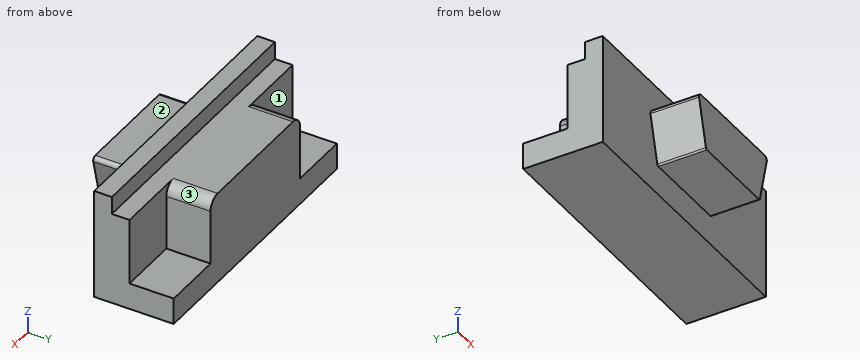
from build123d import *

# Parameters (mm, degrees)
SKETCH008_W          = 30.8
SKETCH008_H          = 12.5
PAD006_DEPTH         = 2
SKETCH009_W          = 30.8
SKETCH009_H          = 10.5
PAD007_DEPTH         = 2
PAD067_DEPTH         = 5
PAD115_DEPTH         = 5.5
BODY_PLACEMENT_ANGLE = 180


with BuildPart() as part:
    # Sketch008 → Pad006 (new body)
    with BuildSketch(Plane(origin=(0, 3, 0), x_dir=(-1, 0, 0), z_dir=(0, 1, 0))):
        with Locations((0, 6.25)):
            Rectangle(SKETCH008_W, SKETCH008_H)
    extrude(amount=-PAD006_DEPTH)

    # Sketch009 → Pad007 (join)
    with BuildSketch(Plane.XZ.offset(-1)):
        with Locations((0, 5.25)):
            Rectangle(SKETCH009_W, SKETCH009_H)
    extrude(amount=PAD007_DEPTH)

    # Sketch010 → Pad067 (join)
    with BuildSketch(Plane.XZ.offset(1)):
        with BuildLine():
            Line((15.4, 0), (15.4, 3))
            Line((15.4, 3), (8.45, 3))
            Line((8.45, 3), (8.45, 9.167398))
            ThreePointArc((8.45, 9.167398), (8.05969, 10.10969), (7.117398, 10.5))
            Line((7.117398, 10.5), (-7.117398, 10.5))
            ThreePointArc((-7.117398, 10.5), (-8.05969, 10.10969), (-8.45, 9.167398))
            Line((-8.45, 9.167398), (-8.45, 3))
            Line((-8.45, 3), (-15.4, 3))
            Line((-15.4, 3), (-15.4, 0))
            Line((-15.4, 0), (15.4, 0))
        make_face()
    extrude(amount=PAD067_DEPTH)

    # Sketch094 → Pad115 (join)
    with BuildSketch(Plane(origin=(0, 3, 0), x_dir=(-1, 0, 0), z_dir=(0, 1, 0))):
        with BuildLine():
            Line((-6, 9.18), (6, 9.18))
            ThreePointArc((6.390856, 8.68), (6.31732, 9.025285), (6, 9.18))
            Line((6.390856, 8.68), (5.098578, 3.485231))
            ThreePointArc((4.9, 3.33), (5.026026, 3.373413), (5.098578, 3.485231))
            Line((4.9, 3.33), (-4.9, 3.33))
            ThreePointArc((-5.098578, 3.485231), (-5.026026, 3.373413), (-4.9, 3.33))
            Line((-5.098578, 3.485231), (-6.390856, 8.68))
            ThreePointArc((-6, 9.18), (-6.31732, 9.025285), (-6.390856, 8.68))
        make_face()
    extrude(amount=PAD115_DEPTH)


with BuildPart() as part_1:
    # Body placement: moved
    add(part.part.moved(Location((5.3, 0, 0))).rotate(Axis((5.3, 0, 0), (0, 0, 1)), BODY_PLACEMENT_ANGLE))


solid = part_1.part
Geometry: final body of the model. Coordinates: model frame, mm. Face numbers are marked on the shaded views. A direction names the side the tool comes from. Coordinates: 2 decimals unless noted, no trailing zeros. Order: outer loops, then holes, each group sorted by start corner. A loop starts at its lowest first (then second) coordinate and runs counter-clockwise, first axis right, second up. Notation, with made-up numbers: (49.25, 33.25) - (67.25, 33.25) arc R18 cw to (67.25, 58.25) - close; hole circle Ø11 at (50, -21). An arc over 180 degrees is marked (long way). Use one line per item in the form item = value.
1) Section B-B (x = 5.5). Return loops of the section in (y, z), then the cut area to 3 significant figures.
Solutions:
outline = (-8.5, 3.33) - (-3, 3.33) - (-3, 0) - (6, 0) - (6, 10.5) - (-1, 10.5) - (-1, 12.5) - (-3, 12.5) - (-3, 9.18) - (-8.5, 9.18) - close
area = 131 mm^2
2) Set-up query: the marked faces 1, 2 and 3. Return all of +Z, -Z, +X, -X, +Y, -Y with unobstructed straight access to the full face (end or side cutting, diameter ignored); none if empty.
Solutions:
face_1 = +Z, -X, +Y
face_2 = +Z, +X, -X, -Y
face_3 = +Z, +X, +Y
3) Section D-D (y = -7). Return loops of the section in (x, z), then the cut area to 3 significant figures.
Solutions:
outline = (-1.09, 8.68) - (0.2, 3.49) arc R0.2 ccw to (0.4, 3.33) - (10.2, 3.33) arc R0.2 ccw to (10.4, 3.49) - (11.69, 8.68) arc R0.4 ccw to (11.3, 9.18) - (-0.7, 9.18) arc R0.4 ccw to start
area = 67.6 mm^2
4) Section A-A (y = 4). Return loops of the section in (x, z).
Solutions:
outline = (-10.1, 0) - (20.7, 0) - (20.7, 3) - (13.75, 3) - (13.75, 9.17) arc R1.33 ccw to (12.42, 10.5) - (-1.82, 10.5) arc R1.33 ccw to (-3.15, 9.17) - (-3.15, 3) - (-10.1, 3) - close
5) Pin query (flat end, axial travel): pin 1 (0.6 mm diameter, centred on x = 7, z = 11.5, fed in from +Y); pin 2 (1.7 mm diameter, centred on x = 5.5, y = -5, fed in from +Z); pin 3 (6 mm diameter, centred on x = 7, y = -6.5, fed in from -Z). Return the tip coordinate at first contact, or that it passes through.
Solutions:
pin_1 = -1
pin_2 = 9.18
pin_3 = 3.33
6) Ray query, L1, parallel to Y at x = -5, z = 4.5; L2, parallel to Z at x = -3.5, y = 1.25; L3, parallel to Y at x = -3, z = 4. Return the intervals inside material, ascending.
Solutions:
L1 = -3 to 1
L2 = 0 to 3
L3 = -3 to 6
7) Section C-C (z = 4.25). Return loops of the section in (x, y), then the cut area to 3 significant figures.
Solutions:
outline = (-10.1, -3) - (0.01, -3) - (0.01, -8.5) - (10.59, -8.5) - (10.59, -3) - (20.7, -3) - (20.7, 1) - (13.75, 1) - (13.75, 6) - (-3.15, 6) - (-3.15, 1) - (-10.1, 1) - close
area = 266 mm^2
